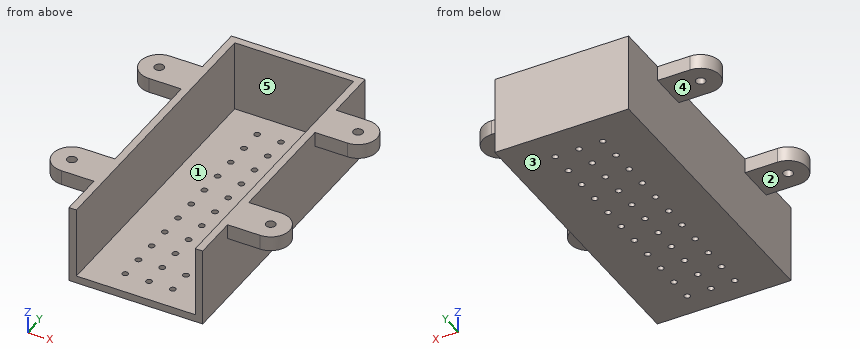
Autodesk Inventor part; units mm, degrees
ref_plane "YZ Plane" through (0, 0, 0) normal (1, 0, 0) x (0, 1, 0)
ref_plane "XZ Plane" through (0, 0, 0) normal (0, 1, 0) x (-1, 0, 0)
ref_plane "XY Plane" through (0, 0, 0) normal (0, 0, 1) x (1, 0, 0)
sketch "Sketch1" plane through (0, 0, 0) normal (0, 0, 1) x (1, 0, 0)
  line L0 (31.75, -76.2) -> (31.75, 76.2)
  line L1 (31.75, 76.2) -> (-31.75, 76.2)
  line L2 (-31.75, 76.2) -> (-31.75, -76.2)
  line L3 (-31.75, -76.2) -> (31.75, 76.2) construction
  line L4 (31.75, -76.2) -> (-31.75, 76.2) construction
  line L5 (35.7188, -76.2) -> (35.7187, 80.1687)
  line L6 (35.7187, 80.1687) -> (-35.7187, 80.1688)
  line L7 (-35.7187, 80.1688) -> (-35.7187, -76.2)
  line L8 (-33.7758, -75.8079) -> (35.7187, 80.1687) construction
  line L9 (33.7758, -75.8079) -> (-35.7187, 80.1688) construction
  line L10 (-31.75, -76.2) -> (-35.7187, -76.2)
  line L11 (31.75, -76.2) -> (35.7188, -76.2)
  point P0 (0, 0)
  dimension "d2" = 3.9688
  dimension "d3" = 3.9688
  dimension "d6" = 152.4
  dimension "d37" = 31.75
  dimension "d38" = 31.75
  dimension "d39" = 3.9688
extrude "Extrusion1" add sketch "Sketch1" along normal blind 38.1
sketch "Sketch2" plane through (0, 0, 0) normal (0, 0, -1) x (-1, 0, 0)
  line L0 (-35.7188, -76.2) -> (-35.7187, 80.1687)
  line L1 (35.7187, 80.1688) -> (35.7187, -76.2)
  line L2 (-35.7187, 80.1687) -> (35.7187, 80.1687)
  line L3 (35.7187, 80.1687) -> (35.7187, -76.2)
  line L4 (35.7187, -76.2) -> (-35.7187, -76.2)
  line L5 (-35.7187, -76.2) -> (-35.7187, 80.1687)
  point P0 (0, 0)
extrude "Extrusion2" add sketch "Sketch2" along normal blind 3.9688
sketch "Sketch5" plane through (0, 0, 38.1) normal (0, 0, 1) x (1, 0, 0)
  line L0 (-35.7187, 80.1688) -> (-35.7187, -76.2)
  line L1 (-35.7187, 42.0688) -> (-53.1074, 42.0688) construction
  line L2 (-35.7187, 31.9088) -> (-53.1074, 31.9088)
  line L3 (-53.1074, 52.2288) -> (-35.7187, 52.2288)
  arc A0 (-53.1074, 52.2288) -> (-53.1074, 31.9088) centre (-53.1074, 42.0688) ccw
  line L4 (35.7187, 80.1687) -> (-35.7187, 80.1688)
  circle A1 centre (-53.1074, 42.0688) radius 2.54
  point P0 (0, 0)
  dimension "d18" = 10.16
  dimension "d21" = 5.08
extrude "Extrusion4" add sketch "Sketch5" against normal blind 7.9375
mirror "Mirror1" about plane through (0, 0, 0) normal (1, 0, 0) of "Extrusion4"
mirror "Mirror2" about plane through (0, 0, 0) normal (0, 1, 0) of "Extrusion4", "Mirror1"
sketch "Sketch6" plane through (0, 0, 0) normal (0, 0, 1) x (1, 0, 0)
  circle A0 centre (-12.7, -63.5) radius 1.5875
  line L0 (-31.75, -76.2) -> (-31.75, 76.2)
  line L1 (-31.75, -76.2) -> (31.75, -76.2) construction
  line L2 (-12.7, -63.5) -> (-12.7, 76.2) construction
  line L3 (-31.75, 76.2) -> (31.75, 76.2) construction
  line L4 (-12.7, -63.5) -> (25.4, -63.5) construction
  circle A1 centre (-12.7, -50.8) radius 1.5875
  circle A2 centre (-12.7, -38.1) radius 1.5875
  circle A3 centre (-12.7, -25.4) radius 1.5875
  circle A4 centre (-12.7, -12.7) radius 1.5875
  circle A5 centre (-12.7, 0) radius 1.5875
  circle A6 centre (-12.7, 12.7) radius 1.5875
  circle A7 centre (-12.7, 25.4) radius 1.5875
  circle A8 centre (-12.7, 38.1) radius 1.5875
  circle A9 centre (-12.7, 50.8) radius 1.5875
  circle A10 centre (-12.7, 63.5) radius 1.5875
  circle A11 centre (0, -63.5) radius 1.5875
  circle A12 centre (0, -50.8) radius 1.5875
  circle A13 centre (0, -38.1) radius 1.5875
  circle A14 centre (0, -25.4) radius 1.5875
  circle A15 centre (0, -12.7) radius 1.5875
  circle A16 centre (0, 0) radius 1.5875
  circle A17 centre (0, 12.7) radius 1.5875
  circle A18 centre (0, 25.4) radius 1.5875
  circle A19 centre (0, 38.1) radius 1.5875
  circle A20 centre (0, 50.8) radius 1.5875
  circle A21 centre (0, 63.5) radius 1.5875
  circle A22 centre (12.7, -63.5) radius 1.5875
  circle A23 centre (12.7, -50.8) radius 1.5875
  circle A24 centre (12.7, -38.1) radius 1.5875
  circle A25 centre (12.7, -25.4) radius 1.5875
  circle A26 centre (12.7, -12.7) radius 1.5875
  circle A27 centre (12.7, 0) radius 1.5875
  circle A28 centre (12.7, 12.7) radius 1.5875
  circle A29 centre (12.7, 25.4) radius 1.5875
  circle A30 centre (12.7, 38.1) radius 1.5875
  circle A31 centre (12.7, 50.8) radius 1.5875
  circle A32 centre (12.7, 63.5) radius 1.5875
  point P0 (0, 0)
  dimension "d24" = 3.175
  dimension "d25" = 19.05
  dimension "d26" = 12.7
  dimension "d29" = 12.7
  dimension "d32" = 12.7
extrude "Extrusion5" cut sketch "Sketch6" against normal through all
sketch "Sketch7" plane through (0, 0, 0) normal (0, 0, 1) x (1, 0, 0)
  point P0 (0, 0)
equation "\"d2\" = wallThickness"
equation "\"d3\" = wallThickness"
equation "\"d6\" = interiorHeight"
equation "\"d39\" = wallThickness"
equation "\"d7\" = interiorDepth"
equation "\"d9\" = wallThickness"
equation "\"d18\" = tabWidth"
equation "\"d21\" = screwHole"
equation "\"d22\" = 2 * wallThickness"
equation "\"interiorWidth\" = 63.5"
equation "\"interiorHeight\" = 152.4"
equation "\"wallThickness\" = 3.96875"
equation "\"interiorDepth\" = 38.1"
equation "\"screwHole\" = 5.08"
equation "\"tabWidth\" = 10.16"
properties part number "thermometerCover"
The model under review builds one solid part; all positions refer to its coordinate system, in mm. Face numbers are marked on the shaded views. A direction names the side the tool comes from. Round coordinates to 2 decimals unless told otherwise and drop trailing zeros. Write each loop counter-clockwise with the first axis right and the second up, starting at its lowest first coordinate (ties: lowest second). Pieces come first, ordered by that corner, then holes. Notation, with made-up numbers: M -16,-36.5 L -10,-36.5 A9 ccw -10,-27.5 Z; hole C 16.25,48.25 d6. An arc over 180 degrees is marked long. Use CSV: the item, a comma, the result in double quotes. Start each with the question number.
(1) Clearance check with flat-ended pins moving along their axes: P1, Ø6, axis at x = -3, y = -59, coming from the +Z side; P2, Ø6, axis at x = -48.5, y = -30, coming from the -Z side; P3, Ø8.5, axis at x = -47, z = 36, coming from the +Y side. State where each tip first meets the part, or that it passes through.
(2) Tool access review of the marked faces 3, 4 and 5: name each direction out of +Z, -Z, +X, -X, +Y, -Y from which nothing blocks a thin tool from reaching the whole face with its end or side.
(3) We need section B-B, the plane z = 19. State the section outline as (x, y) points, then the cut area to 3 significant figures.
(4) We need section D-D, the plane x = -21. State the section outline as (y, z) points.
(5) We need section C-C, the plane y = 57.5. State the section outline as (x, z) points, then the cut area to 3 significant figures.
(6) The part is to be moulded in two halves that separate along X. For the marked faces 1 and 2, say which applies: +X half, -X half, draft (parallel to the pull), parting line (faces both ways), or undercut.
(7) We need section A-A, the plane x = -45. State the section outline as (y, z) points, then the cut area to 3 significant figures.
(8) For line 1 along X through (y, z) = (-50.5, 10.5); line 2 along X through (y, z) = (-25.5, -2); line 3 along X through (y, z) = (-25, -2), list the stretches that pass through material, from the lowest coordinate up.
Findings:
1,P1,"z = 0"
1,P2,"z = 30.16"
1,P3,"y = 52.23"
2,face 3,"-Z, +X, -X, +Y, -Y"
2,face 4,"-Z, -X, +Y, -Y"
2,face 5,"+Z, -Y"
3,outline,"M -35.72,-76.2 L -31.75,-76.2 L -31.75,76.2 L 31.75,76.2 L 31.75,-76.2 L 35.72,-76.2 L 35.72,80.17 L -35.72,80.17 Z"
3,area,"1,490 mm^2"
4,outline,"M -76.2,-3.97 L 80.17,-3.97 L 80.17,38.1 L 76.2,38.1 L 76.2,0 L -76.2,0 Z"
5,outline,"M -35.72,-3.97 L 35.72,-3.97 L 35.72,38.1 L 31.75,38.1 L 31.75,0 L -31.75,0 L -31.75,38.1 L -35.72,38.1 Z"
5,area,"586 mm^2"
6,face 1,"undercut"
6,face 2,"draft"
7,outline,"M -52.23,30.16 L -31.91,30.16 L -31.91,38.1 L -52.23,38.1 Z; M 31.91,30.16 L 52.23,30.16 L 52.23,38.1 L 31.91,38.1 Z"
7,area,"323 mm^2"
8,line 1,"-35.72 to -31.75, 31.75 to 35.72"
8,line 2,"-35.72 to -14.28, -11.12 to -1.58, 1.58 to 11.12, 14.28 to 35.72"
8,line 3,"-35.72 to -14.24, -11.16 to -1.54, 1.54 to 11.16, 14.24 to 35.72"
